The listing builds one solid part. Answer for the finished solid, in the listing's coordinates (mm). A direction names the side the tool comes from. Give positions to 0.01 mm unless a question says otherwise; leave off trailing zeros. Loops run counter-clockwise (first coordinate to the right, second up) from the corner with the lowest first, then second, coordinate; pieces in that order, holes last. Notation, with made-up numbers: (-26.5, 87.25) - (25.5, 87.25) arc R23 ccw to (25.5, 126.25) - close; hole circle Ø5 at (-27, -40). An arc over 180 degrees is marked (long way). Write each question's results on one line, items separated by ' | '.
from build123d import *

# Parameters (mm, degrees)
SKETCH1_W           = 63.5
SKETCH1_H           = 50.8
SKETCH1_R           = 6
BOSS_EXTRUDE1_DEPTH = 3
SKETCH2_W           = 2
SKETCH2_H           = 50.8
BOSS_EXTRUDE2_DEPTH = 24.082
SKETCH3_W           = 8.4
SKETCH3_H           = 8.4
CUT_EXTRUDE1_DEPTH  = 2


with BuildPart() as part:
    # Sketch1 → Boss-Extrude1 (new body)
    with BuildSketch(Plane.XY):
        Rectangle(SKETCH1_W, SKETCH1_H)
        Circle(SKETCH1_R, mode=Mode.SUBTRACT)
    extrude(amount=BOSS_EXTRUDE1_DEPTH)

    # Sketch2 → Boss-Extrude2 (add)
    with BuildSketch(Plane.XY.offset(3)):
        with Locations((-30.75, 0)):
            Rectangle(SKETCH2_W, SKETCH2_H)
    extrude(amount=BOSS_EXTRUDE2_DEPTH)

    # Sketch3 → Cut-Extrude1 (cut)
    with BuildSketch(Plane.ZY.offset(31.75)):
        with Locations((15.8, -0.009)):
            Rectangle(SKETCH3_W, SKETCH3_H)
    extrude(amount=-CUT_EXTRUDE1_DEPTH, mode=Mode.SUBTRACT)


solid = part.part
Item 1: For a pull along Y with two mould halves and no side action, classify faces 4 (the face through (31.75, 0, 1)), 5 (the face through (-7, 25.4, 2)), 6 (the face through (-31, 0, 11.6)) as released by +Y, released by -Y, zero draft, split by the parting line, or undercut.
Values found:
face 4: zero draft | face 5: released by +Y | face 6: undercut
Item 2: For faces 1 (the face through (-29.75, -0.4, 20.2)), 2 (the face through (-31.75, 0, 10)), 3 (the face through (-31, 0, 20)), determine the directions among +Z, -Z, +X, -X, +Y, -Y from which every point of the face is accessible in a straight line to the end or side of a thin tool.
Values found:
face 1: +Z, +X, +Y, -Y | face 2: +Z, -Z, -X, +Y, -Y | face 3: +X, -X
Item 3: A cutting plane is placed at C-C, the plane y = 17. Determine the outline of the cut face in (x, z), plus the area to 3 significant figures.
Values found:
outline: (-31.75, 0) - (31.75, 0) - (31.75, 3) - (-29.75, 3) - (-29.75, 27.08) - (-31.75, 27.08) - close | area: 239 mm²
Item 4: A cutting plane is placed at B-B, the plane x = 0. Determine the outline of the cut face in (y, z), plus the area to 3 significant figures.
Values found:
outline: (-25.4, 0) - (-6, 0) - (-6, 3) - (-25.4, 3) - close; (6, 0) - (25.4, 0) - (25.4, 3) - (6, 3) - close | area: 116 mm²
Item 5: Flat-ended cylindrical pins translate along their axes: P1, Ø3, axis at y = 14, z = 17.5, coming from the +X side; P2, Ø5, axis at x = -18, y = 0.5, coming from the +Z side; P3, Ø4, axis at x = -8.5, y = 2, coming from the -Z side. Find the tip coordinate at first contact, or state that the pin passes through.
Values found:
P1: stops at x = -29.75 | P2: stops at z = 3 | P3: stops at z = 0
Item 6: Find the intervals of material crossed by line 1 along Y through (x, z) = (0, 2.15); line 2 along Z through (x, y) = (-13, -18.5); line 3 along X through (y, z) = (23.5, 23.75), in increasing order. Write a range as [from, to].
Values found:
line 1: y = [-25.4, -6], [6, 25.4] | line 2: z = [0, 3] | line 3: x = [-31.75, -29.75]
Item 7: A cutting plane is placed at D-D, the plane z = 24.75. Determine the outline of the cut face in (x, y).
Values found:
outline: (-31.75, -25.4) - (-29.75, -25.4) - (-29.75, 25.4) - (-31.75, 25.4) - close
Item 8: A cutting plane is placed at A-A, the plane y = 0. Determine the outline of the cut face in (x, z), plus the area to 3 significant figures.
Values found:
outline: (-31.75, 0) - (-6, 0) - (-6, 3) - (-29.75, 3) - (-29.75, 11.6) - (-31.75, 11.6) - close; (-31.75, 20) - (-29.75, 20) - (-29.75, 27.08) - (-31.75, 27.08) - close; (6, 0) - (31.75, 0) - (31.75, 3) - (6, 3) - close | area: 186 mm²
